Read the model definition and answer for the solid it produces. Units are mm, in the model's axes. Round coordinates to 2 decimals unless told otherwise and drop trailing zeros. Write each loop counter-clockwise with the first axis right and the second up, starting at its lowest first coordinate (ties: lowest second). Pieces come first, ordered by that corner, then holes. Notation, with made-up numbers: (3, -37) - (26, -37) arc R20 ccw to (26, -1) - close; hole circle Ø4 at (10.5, -31). An arc over 180 degrees is marked (long way). Answer as CSV lines item,"result". Start each with the question number.
1) Consider line 1 along Y through (x, z) = (6, 1.05); line 2 along X through (y, z) = (17.5, 1.95); line 3 along Y through (x, z) = (28.5, 2.65). Determine where each line is inside the solid, lowest interval first.
2) Find section D-D on z = 0.9. State how many separate pieces and enclosed holes the cut face has, then the cut area to 3 significant figures.
3) Each of these flat-tipped pins is pushed along its axis until it touches: pin 1 (5.5 mm diameter, centred on x = 6.72, y = 44.99, fed in from +Z); pin 2 (1.5 mm diameter, centred on y = 40.5, z = 0.5, fed in from -X). Where does it stop, or does it pass through?
4) Find section A-A on y = 4. Determine the outline of the cut face in (x, z).
5) Find section C-C on y = 10. Determine the outline of the cut face in (x, z), then the cut area to 3 significant figures.
6) Find section B-B on x = 44. Determine the outline of the cut face in (y, z), then the cut area to 3 significant figures.
from build123d import *

# Parameters (mm, degrees)
EXTRUDE_1_DEPTH     = 3
SKETCH_2_R          = 2.1
CUT_EXTRUDE_1_DEPTH = 10


with BuildPart() as part:
    # 草图1 → 凸台-拉伸1 (new body)
    with BuildSketch(Plane.XY):
        Polygon((60, 0), (0, 0), (0, 20), (20, 20), (-5.980762114, 35), (4.019237886, 52.320508076), (60, 20), align=None)
    extrude(amount=EXTRUDE_1_DEPTH)

    # 草图2 → 切除-拉伸1 (cut)
    with BuildSketch(Plane.XY.offset(3)):
        with Locations((6.715390309, 44.990381057)):
            Circle(SKETCH_2_R)
        with Locations((1.715390309, 36.330127019)):
            Circle(SKETCH_2_R)
        with Locations((17.540707856, 38.740381057)):
            Circle(SKETCH_2_R)
        with Locations((12.540707856, 30.080127019)):
            Circle(SKETCH_2_R)
        with Locations((23.366025404, 23.830127019)):
            Circle(SKETCH_2_R)
        with Locations((28.366025404, 32.490381057)):
            Circle(SKETCH_2_R)
        with Locations((6, 16)):
            Circle(SKETCH_2_R)
        with Locations((6, 4)):
            Circle(SKETCH_2_R)
        with Locations((54, 16)):
            Circle(SKETCH_2_R)
        with Locations((54, 4)):
            Circle(SKETCH_2_R)
        with Locations((16, 16)):
            Circle(SKETCH_2_R)
        with Locations((16, 4)):
            Circle(SKETCH_2_R)
        with Locations((44, 16)):
            Circle(SKETCH_2_R)
        with Locations((44, 4)):
            Circle(SKETCH_2_R)
        with BuildLine():
            Line((21, 14), (39, 14))
            ThreePointArc((39, 14), (43, 10), (39, 6))
            Line((39, 6), (21, 6))
            ThreePointArc((21, 6), (17, 10), (21, 14))
        make_face()
    extrude(amount=-CUT_EXTRUDE_1_DEPTH, mode=Mode.SUBTRACT)


solid = part.part
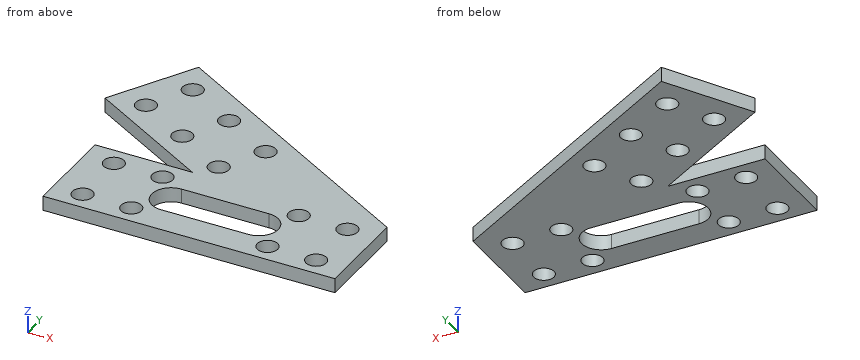
Check values:
1,line 1,"y = 0 to 1.9, 6.1 to 13.9, 18.1 to 20, 28.08 to 43.02, 46.96 to 51.18"
1,line 2,"x = 0 to 4.53, 7.47 to 14.53, 17.47 to 42.53, 45.47 to 52.53, 55.47 to 60"
1,line 3,"y = 0 to 6, 14 to 30.39, 34.59 to 38.19"
2,separate pieces,"1"
2,enclosed holes,"15"
2,area,"1,760 mm^2"
3,pin 1,"stops at z = 3"
3,pin 2,"stops at x = -3.24"
4,outline,"(0, 0) - (3.9, 0) - (3.9, 3) - (0, 3) - close; (8.1, 0) - (13.9, 0) - (13.9, 3) - (8.1, 3) - close; (18.1, 0) - (41.9, 0) - (41.9, 3) - (18.1, 3) - close; (46.1, 0) - (51.9, 0) - (51.9, 3) - (46.1, 3) - close; (56.1, 0) - (60, 0) - (60, 3) - (56.1, 3) - close"
5,outline,"(0, 0) - (17, 0) - (17, 3) - (0, 3) - close; (43, 0) - (60, 0) - (60, 3) - (43, 3) - close"
5,area,"102 mm^2"
6,outline,"(0, 0) - (1.9, 0) - (1.9, 3) - (0, 3) - close; (6.1, 0) - (13.9, 0) - (13.9, 3) - (6.1, 3) - close; (18.1, 0) - (29.24, 0) - (29.24, 3) - (18.1, 3) - close"
6,area,"62.5 mm^2"
